Autodesk Inventor part; units mm, degrees
ref_plane "YZ Plane" through (0, 0, 0) normal (1, 0, 0) x (0, 1, 0)
ref_plane "XZ Plane" through (0, 0, 0) normal (0, 1, 0) x (-1, 0, 0)
ref_plane "XY Plane" through (0, 0, 0) normal (0, 0, 1) x (1, 0, 0)
sketch "Szkic1" plane through (0, 0, 0) normal (0, 1, 0) x (-1, 0, 0)
  line L0 (-19.5, -35.5) -> (19.5, -35.5)
  line L1 (19.5, -35.5) -> (19.5, 35.5)
  line L2 (19.5, 35.5) -> (-19.5, 35.5)
  line L3 (-19.5, 35.5) -> (-19.5, -35.5)
  line L4 (-19.5, -35.5) -> (19.5, 35.5) construction
  line L5 (19.5, -35.5) -> (-19.5, 35.5) construction
  point P0 (0, 0)
  dimension "d0" = 39
  dimension "d1" = 71
extrude "Wyciągnięcie proste1" add sketch "Szkic1" along normal blind 4
sketch "Szkic2" plane through (0, 4, 0) normal (0, 1, 0) x (1, 0, 0)
  line L0 (19.5, 35.5) -> (-19.5, 35.5)
  line L1 (-19.5, 35.5) -> (-19.5, -35.5)
  line L2 (-19.5, -35.5) -> (19.5, -35.5)
  line L3 (19.5, -35.5) -> (19.5, 35.5)
  point P0 (0, 0)
  point P1 (-15, -31.5)
  point P2 (-15, 31.5)
  point P3 (15, 31.5)
  point P4 (15, -31.5)
  point P5 (-15, 0)
  point P6 (7, 0)
  dimension "d4" = 4
  dimension "d5" = 4.5
  dimension "d6" = 63
  dimension "d7" = 63
  dimension "d8" = 71
  dimension "d9" = 4
  dimension "d10" = 30
  dimension "d11" = 39
  dimension "d12" = 30
  dimension "d13" = 4.5
  dimension "d29" = 4.5
  dimension "d30" = 31.5
  dimension "d31" = 22
hole "Otwór1" at (-15, 4, 31.5) at (-15, 4, -31.5) at (15, 4, -31.5) at (15, 4, 31.5) at (7, 4, 0) at (-15, 4, 0) direction (0, -1, 0) diameter 3 end through all
sketch "Szkic3" plane through (0, 4, 0) normal (0, 1, 0) x (1, 0, 0)
  circle A0 centre (15, 31.5) radius 1.5
  circle A1 centre (-15, -31.5) radius 1.5
  circle A2 centre (-15, 31.5) radius 1.5
  circle A3 centre (15, -31.5) radius 1.5
  line L0 (19.5, 35.5) -> (-19.5, 35.5)
  line L1 (-19.5, 35.5) -> (-19.5, -35.5)
  line L2 (-19.5, -35.5) -> (19.5, -35.5)
  line L3 (19.5, -35.5) -> (19.5, 35.5)
  line L4 (12.5, -26.5) -> (19.5, -26.5)
  line L5 (19.5, -26.5) -> (19.5, 3.5)
  line L6 (19.5, 3.5) -> (12.5, 3.5)
  line L7 (12.5, 3.5) -> (12.5, -26.5)
  point P0 (0, 0)
  dimension "d21" = 7
  dimension "d22" = 30
  dimension "d23" = 0
  dimension "d24" = 9
extrude "Wyciągnięcie proste2" add sketch "Szkic3" along normal blind 10 contours L3 L4 L7 L6
sketch "Szkic4" plane through (19.5, 0, 35.5) normal (1, 0, 0) x (0, 0, -1)
  line L0 (0, 0) -> (71, 0)
  line L1 (71, 0) -> (71, 4)
  line L2 (39, 4) -> (71, 4)
  line L3 (39, 4) -> (39, 14)
  line L4 (9, 14) -> (39, 14)
  line L5 (9, 4) -> (9, 14)
  line L6 (0, 4) -> (9, 4)
  line L7 (0, 0) -> (0, 4)
  line L8 (9, 14) -> (39, 14)
  line L9 (39, 14) -> (39, 4)
  line L10 (39, 4) -> (9, 4)
  line L11 (9, 4) -> (9, 14)
  point P0 (35.5, 0)
extrude "Wyciągnięcie proste3" add sketch "Szkic4" along normal blind 15 contours L5 L4 L3 L10
properties part number "MostekH"
The listing builds one solid part. Answer for the finished solid, in the listing's coordinates (mm). A direction names the side the tool comes from. Give positions to 0.01 mm unless a question says otherwise; leave off trailing zeros. Loops run counter-clockwise (first coordinate to the right, second up) from the corner with the lowest first, then second, coordinate; pieces in that order, holes last. Notation, with made-up numbers: (81.25, -9.5) - (132.25, -9.5) arc R24 cw to (132.25, 17.5) - close; hole circle Ø2 at (-4, 27.25). An arc over 180 degrees is marked (long way). Answer as a JSON object with one key per item and string values.
1. A cutting plane is placed at B-B (z = -31.5). Write down the section's boundary in (x, y).
Determined:
{"outline": "(-19.5, 0) - (-16.5, 0) - (-16.5, 4) - (-19.5, 4) - close; (-13.5, 0) - (13.5, 0) - (13.5, 4) - (-13.5, 4) - close; (16.5, 0) - (19.5, 0) - (19.5, 4) - (16.5, 4) - close"}
2. For a pull along X with two mould halves and no side action, classify faces 5 (the flat face through (0, 2, 35.5)), 6 (the cylindrical face through (15.9, 2, -32.7)), 7 (the flat face through (34.5, 9, 12)), 8 (the cylindrical face through (-16.01, 1.97, -1.11)) as pulls with the +X half, pulls with the -X half, needs draft (parallel to the pull), parting line crosses it, or undercut.
Determined:
{"face 5": "needs draft", "face 6": "undercut", "face 7": "pulls with the +X half", "face 8": "undercut"}
3. A cutting plane is placed at C-C (x = 15). Write down the section's boundary in (y, z), then the cut area to 3 significant figures.
Determined:
{"outline": "(0, -35.5) - (4, -35.5) - (4, -33) - (0, -33) - close; (0, -30) - (4, -30) - (4, -3.5) - (14, -3.5) - (14, 26.5) - (4, 26.5) - (4, 30) - (0, 30) - close; (0, 33) - (4, 33) - (4, 35.5) - (0, 35.5) - close", "area": "560 mm²"}
4. Find the intervals of material crossed by L1, parallel to X at y = 2.65, z = -31.5; L2, parallel to X at y = 1.7, z = 0; L3, parallel to Z at x = 15, y = 2.05, in increasing order. Write a range as [from, to].
Determined:
{"L1": "[-19.5, -16.5], [-13.5, 13.5], [16.5, 19.5]", "L2": "[-19.5, -16.5], [-13.5, 5.5], [8.5, 19.5]", "L3": "[-35.5, -33], [-30, 30], [33, 35.5]"}
5. Flat-ended cylindrical pins translate along their axes: pin 1 Ø4.5 at (y, z) = (2.5, -11.5) entering from +X; pin 2 Ø2 at (x, z) = (2.5, -23.5) entering from +Y; pin 3 Ø1.8 at (x, z) = (-15, 31.5) entering from -Y; pin 4 Ø7.5 at (x, z) = (25.5, 9) entering from -Y. Find the tip coordinate at first contact, or state that the pin passes through.
Determined:
{"pin 1": "x = 19.5", "pin 2": "y = 4", "pin 3": "through", "pin 4": "y = 4"}
6. For faces 1 (the flat face through (27, 4, 11)), 2 (the flat face through (23, 9, 26.5)), 3 (the flat face through (12.5, 9, 11)), 4 (the flat face through (23, 9, -3.5)), determine the directions among +Z, -Z, +X, -X, +Y, -Y from which every point of the face is accessible in a straight line to the end or side of a thin tool.
Determined:
{"face 1": "+Z, -Z, +X, -Y", "face 2": "+Z, +X, -X, +Y", "face 3": "+Z, -Z, -X, +Y", "face 4": "-Z, +X, -X, +Y"}
7. A cutting plane is placed at D-D (y = 1). Write down the section's boundary in (x, z), then the cut area to 3 significant figures.
Determined:
{"outline": "(-19.5, -35.5) - (19.5, -35.5) - (19.5, 35.5) - (-19.5, 35.5) - close; hole circle Ø3 at (-15, -31.5); hole circle Ø3 at (-15, 0); hole circle Ø3 at (-15, 31.5); hole circle Ø3 at (7, 0); hole circle Ø3 at (15, -31.5); hole circle Ø3 at (15, 31.5)", "area": "2,730 mm²"}
8. A cutting plane is placed at A-A (x = 7). Write down the section's boundary in (y, z).
Determined:
{"outline": "(0, -35.5) - (4, -35.5) - (4, -1.5) - (0, -1.5) - close; (0, 1.5) - (4, 1.5) - (4, 35.5) - (0, 35.5) - close"}
